Input: part model. Units: mm. Frame: model coordinates. Round coordinates to 2 decimals unless told otherwise and drop trailing zeros. Loops run counter-clockwise (first coordinate to the right, second up) from the corner with the lowest first, then second, coordinate; pieces in that order, holes last. Notation, with made-up numbers: M 72,42 L 125,42 A17 ccw 125,51 Z; hole C 30.5,-33 d10. An arc over 180 degrees is marked long. Return JSON: item names as keys, results as strings. Group by question number.
1) Material intervals for line 1 (Y direction, x = 0, z = 0.15); line 2 (Y direction, x = -1, z = -0.8); line 3 (X direction, y = -0.75, z = 0.35), sorted ascending. Write a range as from..to.
2) Mould query, pull axis X, two halves, no side actions, for faces 1 (the face through (0, -3.4, 0)), 2 (the face through (2, 0, 0)), 3 (the face through (-2.651, -2.632, 1.166)), 4 (the face through (2.66, 2.64, -1.16)). Classes: +X half, -X half, draft (parallel to the pull), parting line (faces both ways), or undercut.
3) Section A-A (z = -0.25). Output: boundary loops of the cut face in (x, y).
from build123d import *

# Parameters (mm, degrees)
SKETCH2_OUTSIDE_W   = 14.88
SKETCH2_OUTSIDE_H   = 14.88
SKETCH2_OUTSIDE_W_2 = 6.8
SKETCH2_OUTSIDE_H_2 = 6.8
CUT_EXTRUDE1_DEPTH  = 1.36


with BuildPart() as part:
    # Sketch1 → Revolve1 (revolve)
    with BuildSketch(Plane(origin=(0, 0, 0), x_dir=(0, 0, -1), z_dir=(1, 0, 0))):
        Polygon((0.436239569, 5), (-0.436239569, 5), (-1.36, 3.4), (-1.36, 2.36), (-1.107925286, 2), (1.107925286, 2), (1.36, 2.36), (1.36, 3.4), align=None)
    revolve(axis=Axis((0, 0, -2), (0, 0, 1)))

    # Sketch2 outside → Cut-Extrude1 (cut, symmetric)
    with BuildSketch(Plane.XY):
        Rectangle(SKETCH2_OUTSIDE_W, SKETCH2_OUTSIDE_H)
        Rectangle(SKETCH2_OUTSIDE_W_2, SKETCH2_OUTSIDE_H_2, mode=Mode.SUBTRACT)
    extrude(amount=CUT_EXTRUDE1_DEPTH, both=True, mode=Mode.SUBTRACT)


solid = part.part
Returned:
{
 "1": {"line 1": "y = -3.4..-2, 2..3.4", "line 2": "y = -3.4..-1.73, 1.73..3.4", "line 3": "x = -3.4..-1.85, 1.85..3.4"},
 "2": {"face 1": "draft", "face 2": "undercut", "face 3": "-X half", "face 4": "+X half"},
 "3": {"outline": "M -3.4,-3.4 L 3.4,-3.4 L 3.4,3.4 L -3.4,3.4 Z; hole C 0,0 d4"}
}
